```python
from build123d import *

# Parameters (mm, degrees)
F1_DEPTH = 508
F2_W     = 19.05
F2_H     = 76.2
F3_DEPTH = 25.4
F4_W     = 76.2
F4_H     = 6.35
F5_DEPTH = 50.801


with BuildPart() as f1:
    # F0 (on Front) → F1 (new body)
    with BuildSketch(Plane.XZ):
        Polygon((0, -19.05), (0, 0), (-50.8, 0), (-31.75, -19.05), align=None)
    extrude(amount=F1_DEPTH)

    # F2 (on face) → F3 (cut)
    with BuildSketch(Plane.XY):
        with Locations((-41.275, -38.1)):
            Rectangle(F2_W, F2_H)
        with Locations((-41.275, -469.9)):
            Rectangle(F2_W, F2_H)
    extrude(amount=-F3_DEPTH, mode=Mode.SUBTRACT)

    # F4 (on face) → F5 (cut, through all)
    with BuildSketch(Plane.YZ):
        with Locations((-469.9, -15.875)):
            Rectangle(F4_W, F4_H)
        with Locations((-38.1, -15.875)):
            Rectangle(F4_W, F4_H)
    extrude(amount=-F5_DEPTH, mode=Mode.SUBTRACT)


solid = f1.part
```
Part model, mm, in its own coordinate system. A direction names the side the tool comes from. Coordinates: 2 decimals unless noted, no trailing zeros. Order: outer loops, then holes, each group sorted by start corner. A loop starts at its lowest first (then second) coordinate and runs counter-clockwise, first axis right, second up. Notation, with made-up numbers: (-27, -1.5) - (-14, -1.5) arc R20 cw to (-14, 8.5) - close; hole circle Ø9 at (63.25, 4). An arc over 180 degrees is marked (long way). Return JSON: item names as keys, results as strings. Group by question number.
Item 1: Pin check, flat tips, straight feed: pin 1 (4 mm diameter, centred on y = -176.5, z = -4.5, fed in from -X); pin 2 (9.5 mm diameter, centred on x = -15, y = -465.5, fed in from -Z); pin 3 (5 mm diameter, centred on y = -216.5, z = -9, fed in from -X). Stop position of each tip, or through.
Item 2: Cut at B-B (z = -7). List the corners of the cut face in (x, y), plus the area to 3 significant figures.
Item 3: Cut at C-C (y = -295). List the corners of the cut face in (x, z).
Item 4: Drill centre lines: probe 1 along X at (y, z) = (-439.5, -3.5); probe 2 along Z at (x, y) = (-29, -58.5); probe 3 along Y at (x, z) = (-38, -3.75). Where is each one in solid material? Low to high. Write a range as from..to.
Item 5: Cut at A-A (x = -11.5). List the corners of the cut face in (y, z).
Item 6: Which spindle directions (+Z, -Z, +X, -X, +Y, -Y) get a long thin tool onto all of the face, cutting with end or side? Do faces 1 (the face through (-31.75, -470, -6)), 2 (the face through (-16, -470, -12.7)), 3 (the face through (-16, -39, -12.7)), 4 (the face through (-16, -508, -6)), 5 (the face through (-31.75, -39, -6)). Say none if no direction does.
Check values:
{
 "1": {"pin 1": "stops at x = -48.3", "pin 2": "stops at z = -12.7", "pin 3": "stops at x = -44.3"},
 "2": {"outline": "(-43.8, -431.8) - (-31.75, -431.8) - (-31.75, -508) - (0, -508) - (0, 0) - (-31.75, 0) - (-31.75, -76.2) - (-43.8, -76.2) - close", "area": "20,400 mm2"},
 "3": {"outline": "(-50.8, 0) - (-31.75, -19.05) - (0, -19.05) - (0, 0) - close"},
 "4": {"probe 1": "x = -31.75..0", "probe 2": "z = -12.7..0", "probe 3": "y = -431.8..-76.2"},
 "5": {"outline": "(-508, -12.7) - (-431.8, -12.7) - (-431.8, -19.05) - (-76.2, -19.05) - (-76.2, -12.7) - (0, -12.7) - (0, 0) - (-508, 0) - close"},
 "6": {"face 1": "+Z, -Z, -X, -Y", "face 2": "-Z, +X, -X, -Y", "face 3": "-Z, +X, -X, +Y", "face 4": "+Z, -Z, +X, -X, -Y", "face 5": "+Z, -Z, -X, +Y"}
}
